```python
from build123d import *

# Parameters (mm, degrees)
EXTRUDE_1_DEPTH              = 9
SKETCH_2_W                   = 20
SKETCH_2_H                   = 8
CUT_EXTRUDE_1_DEPTH          = 5.5
SKETCH_3_W                   = 10
SKETCH_3_H                   = 4
EXTRUDE_2_DEPTH              = 5
HOLE_WIZARD_20_0_20_1_D      = 20
HOLE_WIZARD_20_0_20_1_DEPTH  = 14
HOLE_WIZARD_2_5_2_5_1_D      = 2.5
HOLE_WIZARD_2_5_2_5_1_DEPTH  = 57.5
HOLE_WIZARD_2_5_2_5_2_D      = 2.5
HOLE_WIZARD_2_5_2_5_2_DEPTH  = 4
HOLE_WIZARD_M3_1_D           = 3.2
HOLE_WIZARD_M3_1_CBORE_D     = 6
HOLE_WIZARD_M3_1_CBORE_DEPTH = 5
FILLET_1_R                   = 0.5
FILLET_2_R                   = 1


with BuildPart() as part:
    # 草图1 → 凸台-拉伸1 (new body)
    with BuildSketch(Plane(origin=(0, 0, 0), x_dir=(-1, 0, 0), z_dir=(0, 0, -1))):
        with BuildLine():
            Line((-12, -25.850531909), (-12, -34.5))
            Line((-12, -34.5), (12, -34.5))
            Line((12, -34.5), (12, -25.850531909))
            ThreePointArc((12, -25.850531909), (0, 28.5), (-12, -25.850531909))
        make_face()
    extrude(amount=-EXTRUDE_1_DEPTH)

    # 草图2 → 切除-拉伸1 (cut)
    with BuildSketch(Plane.XZ.offset(34.5)):
        with Locations((0, 5)):
            Rectangle(SKETCH_2_W, SKETCH_2_H)
    extrude(amount=-CUT_EXTRUDE_1_DEPTH, mode=Mode.SUBTRACT)

    # 草图3 → 凸台-拉伸2 (add)
    with BuildSketch(Plane.XY.offset(9)):
        with Locations((0, -27)):
            Rectangle(SKETCH_3_W, SKETCH_3_H)
    extrude(amount=EXTRUDE_2_DEPTH)

    # Ø20.0 (20) 直径孔1
    with Locations(Plane(origin=(0, 0, 0), x_dir=(-1, 0, 0), z_dir=(0, 0, -1))):
        with Locations((0, 0)):
            Hole(HOLE_WIZARD_20_0_20_1_D / 2, depth=HOLE_WIZARD_20_0_20_1_DEPTH)

    # Ø2.5 (2.5) 直径孔1
    with Locations(Plane.XZ.offset(29)):
        with Locations((0, 11.5)):
            Hole(HOLE_WIZARD_2_5_2_5_1_D / 2, depth=HOLE_WIZARD_2_5_2_5_1_DEPTH)

    # Ø2.5 (2.5) 直径孔2
    with Locations(Plane.XZ.offset(29)):
        with Locations((5.5, 5), (-5.5, 5)):
            Hole(HOLE_WIZARD_2_5_2_5_2_D / 2, depth=HOLE_WIZARD_2_5_2_5_2_DEPTH)

    # M3 六角头机械螺钉的柱形沉头孔1 (through all)
    with Locations(Plane.XY.offset(9)):
        with Locations((-13.435028843, -13.435028843), (-13.435028843, 13.435028843), (13.435028843, 13.435028843), (13.435028843, -13.435028843)):
            CounterBoreHole(HOLE_WIZARD_M3_1_D / 2, HOLE_WIZARD_M3_1_CBORE_D / 2, HOLE_WIZARD_M3_1_CBORE_DEPTH)

    # 圆角1
    fillet_1_edges = [part.edges().sort_by_distance(p)[0] for p in [
        (10, -31.75, 1),
        (-10, -31.75, 1),
    ]]
    fillet(fillet_1_edges, radius=FILLET_1_R)

    # 圆角2
    fillet_2_edges = [part.edges().sort_by_distance(p)[0] for p in [
        (5, -27, 9),
        (-5, -27, 9),
        (5, -27, 14),
        (-5, -27, 14),
        (-12, -30.175265955, 0),
        (12, -30.175265955, 0),
    ]]
    fillet(fillet_2_edges, radius=FILLET_2_R)


solid = part.part
```
Model file for the job. Use its own axes, mm. A direction names the side the tool comes from. Coordinates: 2 decimals unless noted, no trailing zeros. Order: outer loops, then holes, each group sorted by start corner. A loop starts at its lowest first (then second) coordinate and runs counter-clockwise, first axis right, second up. Notation, with made-up numbers: (2, 44) -> (39, 44) arc R17 cw to (39, 54) -> close; hole circle Ø9 at (47.25, 22). An arc over 180 degrees is marked (long way). Answer as a JSON object with one key per item and string values. Group by question number.
1) Which spindle directions (+Z, -Z, +X, -X, +Y, -Y) get a long thin tool onto all of the face, cutting with end or side? Do faces 1 (the face through (5, -27, 11)), 2 (the face through (15, 12, 4)), 3 (the face through (5.77, -26.97, 3.78)). Say none if no direction does.
2) Flat gauge pins, fed straight in: pin 1 (2.5 mm diameter, centred on y = -28, z = 11.5, fed in from +X); pin 2 (6 mm diameter, centred on y = -32.5, z = 7, fed in from +X); pin 3 (3 mm diameter, centred on y = 3.5, z = 7, fed in from +X). Where does each tip first touch, or does it go through?
3) Cut at D-D, the plane y = 7.5. Write the cut outline in (x, z), then the cut area to 3 significant figures.
4) Cut at A-A, the plane x = 0. Write the cut outline in (y, z), then the cut area to 3 significant figures.
5) Cut at B-B, the plane y = 0. Write the cut outline in (x, z).
6) Drill centre lines: L1, parallel to X at y = 11, z = 8.25; L2, parallel to X at y = 13.5, z = 5; L3, parallel to Z at x = -6.5, y = -31.5. Where is each one in solid material? Low to high.
7) Cut at C-C, the plane z = 7. Write the cut outline in (x, y), then the cut area to 3 significant figures.
8) Pull direction Z, two halves, no side cores. Call faces 4 (the face through (-12, -15, 4)), 5 (the face through (0.16, -26.97, 12.74)), 6 (the face through (-5, -27, 11)): +Z half, -Z half, draft (parallel to the pull), parting line (faces both ways), or undercut.
Check values:
{
 "1": {"face 1": "+Z, +X, +Y, -Y", "face 2": "+Z", "face 3": "-Y"},
 "2": {"pin 1": "stops at x = 5", "pin 2": "stops at x = 12", "pin 3": "stops at x = 28.43"},
 "3": {"outline": "(-27.5, 0) -> (-6.61, 0) -> (-6.61, 9) -> (-27.5, 9) -> close; (6.61, 0) -> (27.5, 0) -> (27.5, 9) -> (6.61, 9) -> close", "area": "376 mm²"},
 "4": {"outline": "(-34.5, 0) -> (-10, 0) -> (-10, 9) -> (-25, 9) -> (-25, 10.25) -> (-29, 10.25) -> (-29, 1) -> (-34.5, 1) -> close; (-29, 12.75) -> (-25, 12.75) -> (-25, 14) -> (-29, 14) -> close; (10, 0) -> (28.5, 0) -> (28.5, 9) -> (10, 9) -> close", "area": "353 mm²"},
 "5": {"outline": "(-28.5, 0) -> (-10, 0) -> (-10, 9) -> (-28.5, 9) -> close; (10, 0) -> (28.5, 0) -> (28.5, 9) -> (10, 9) -> close"},
 "6": {"L1": "x = -26.29 to -15.19, -11.68 to 11.68, 15.19 to 26.29", "L2": "x = -25.1 to -16.43, -10.44 to 10.44, 16.43 to 25.1", "L3": "z = 0 to 1"},
 "7": {"outline": "(-12, -34.5) -> (-10, -34.5) -> (-10, -29) -> (10, -29) -> (10, -34.5) -> (12, -34.5) -> (12, -25.85) arc R28.5 ccw (long way) to (-12, -25.85) -> close; hole circle Ø6 at (-13.44, -13.44); hole circle Ø6 at (-13.44, 13.44); hole circle Ø20 at (0, 0); hole circle Ø6 at (13.44, -13.44); hole circle Ø6 at (13.44, 13.44)", "area": "2,180 mm²"},
 "8": {"face 4": "+Z half", "face 5": "undercut", "face 6": "draft"}
}
